```python
from build123d import *
from OCP.BRepFilletAPI import BRepFilletAPI_MakeChamfer

# Parameters (mm, degrees)
SKETCH1_W               = 71
SKETCH1_H               = 71
SKETCH1_W_2             = 21
SKETCH1_H_2             = 21
BOSS_EXTRUDE1_DEPTH     = 25
SKETCH2_W               = 21
SKETCH2_H               = 23
BOSS_EXTRUDE2_DEPTH     = 2
CHAMFER1_SIZE           = 2
CHAMFER1_SIZE_2         = 20
CUT_EXTRUDE1_DEPTH      = 84.846586096
CUT_EXTRUDE1_DEPTH_BACK = 5
SKETCH3_R               = 1.5
SKETCH4_R               = 1.5
CUT_EXTRUDE2_DEPTH      = 5
CUT_EXTRUDE3_START      = -5
SKETCH5_R               = 1.5
CUT_EXTRUDE3_DEPTH      = 5
SKETCH6_W               = 21
SKETCH6_H               = 20
SKETCH6_R               = 2.5
CUT_EXTRUDE4_DEPTH      = 21
CUT_EXTRUDE5_DEPTH      = 30
CHAMFER2_SIZE           = 2


with BuildPart() as part:
    # Sketch1 → Boss-Extrude1 (new body)
    with BuildSketch(Plane(origin=(0, 0, 0), x_dir=(1, 0, 0), z_dir=(0, 1, 0))):
        Rectangle(SKETCH1_W, SKETCH1_H)
        Polygon((-13, 9.464466094), (-13, -9.464466094), (-30.5, -26.964466094), (-30.5, 26.964466094), align=None, mode=Mode.SUBTRACT)
        Rectangle(SKETCH1_W_2, SKETCH1_H_2, mode=Mode.SUBTRACT)
        Polygon((30.5, -26.964466094), (13, -9.464466094), (13, 9.464466094), (30.5, 26.964466094), align=None, mode=Mode.SUBTRACT)
        Polygon((9.464466094, 13), (-9.464466094, 13), (-26.964466094, 30.5), (26.964466094, 30.5), align=None, mode=Mode.SUBTRACT)
    extrude(amount=BOSS_EXTRUDE1_DEPTH)

    # Sketch2 → Boss-Extrude2 (add)
    with BuildSketch(Plane(origin=(0, 25, 0), x_dir=(1, 0, 0), z_dir=(0, 1, 0))):
        Polygon((-33.5, -35.5), (-10.5, -35.5), (-10.5, -12.5), align=None)
        with Locations((0, -24)):
            Rectangle(SKETCH2_W, SKETCH2_H)
        Polygon((10.5, -12.5), (10.5, -35.5), (33.5, -35.5), align=None)
    extrude(amount=BOSS_EXTRUDE2_DEPTH)

    # Chamfer1
    chamfer1_edges_1 = [part.edges().sort_by_distance(p)[0] for p in [
        (22, 27, 24),
    ]]
    chamfer1_side_1 = [part.faces().sort_by_distance(p)[0] for p in [
        (22, 26.96, 24),
    ]]
    chamfer1_edges_2 = [part.edges().sort_by_distance(p)[0] for p in [
        (0, 27, 12.5),
    ]]
    chamfer1_side_2 = [part.faces().sort_by_distance(p)[0] for p in [
        (0, 26.96, 12.5),
    ]]
    chamfer1_edges_3 = [part.edges().sort_by_distance(p)[0] for p in [
        (-22, 27, 24),
    ]]
    chamfer1_side_3 = [part.faces().sort_by_distance(p)[0] for p in [
        (-22, 26.96, 24),
    ]]
    chamfer1 = BRepFilletAPI_MakeChamfer(part.part.solid().wrapped)
    for e in chamfer1_edges_1:
        chamfer1.Add(CHAMFER1_SIZE - 0.0001, CHAMFER1_SIZE_2 - 0.0001, e.wrapped, chamfer1_side_1[0].wrapped)
    for e in chamfer1_edges_2:
        chamfer1.Add(CHAMFER1_SIZE - 0.0001, CHAMFER1_SIZE_2 - 0.0001, e.wrapped, chamfer1_side_2[0].wrapped)
    for e in chamfer1_edges_3:
        chamfer1.Add(CHAMFER1_SIZE - 0.0001, CHAMFER1_SIZE_2 - 0.0001, e.wrapped, chamfer1_side_3[0].wrapped)
    add(Compound.cast(chamfer1.Shape()), mode=Mode.REPLACE)  # a hair under: the kernel refuses the full size

    # Sketch3 → Cut-Extrude1 (cut, two sides: drawn at the far end of the back side and taken through both)
    with BuildSketch(Plane.ZY.offset(35.5).offset(-CUT_EXTRUDE1_DEPTH_BACK)):
        with Locations(Location((-10, 12.5, 0), (0, 0, 180))):
            Circle(SKETCH3_R)
        with BuildLine():
            ThreePointArc((0, 14), (-1.5, 12.5), (0, 11))
            Line((0, 11), (0, 14))
        make_face()
        with BuildLine():
            Line((0, 14), (0, 11))
            ThreePointArc((0, 11), (1.060660172, 11.439339828), (1.5, 12.5))
            ThreePointArc((1.5, 12.5), (1.060660172, 13.560660172), (0, 14))
        make_face()
        with Locations(Location((10, 12.5, 0), (0, 0, 180))):
            Circle(SKETCH3_R)
    extrude(amount=CUT_EXTRUDE1_DEPTH + CUT_EXTRUDE1_DEPTH_BACK, mode=Mode.SUBTRACT)

    # Sketch4 → Cut-Extrude2 (cut)
    with BuildSketch(Plane(origin=(0, 0, -35.5), x_dir=(-1, 0, 0), z_dir=(0, 0, -1))):
        with Locations((-10, 12.5)):
            Circle(SKETCH4_R)
        with Locations((0, 12.5)):
            Circle(SKETCH4_R)
        with Locations((10, 12.5)):
            Circle(SKETCH4_R)
    extrude(amount=-CUT_EXTRUDE2_DEPTH, mode=Mode.SUBTRACT)

    # Sketch5 → Cut-Extrude3 (cut)
    with BuildSketch(Plane(origin=(35.5, 0, 0), x_dir=(0, 0, -1), z_dir=(1, 0, 0)).offset(CUT_EXTRUDE3_START)):
        with Locations((-10, 12.5)):
            Circle(SKETCH5_R)
        with BuildLine():
            ThreePointArc((1.5, 12.5), (1.060660172, 13.560660172), (0, 14))
            Line((0, 14), (0, 11))
            ThreePointArc((0, 11), (1.060660172, 11.439339828), (1.5, 12.5))
        make_face()
        with BuildLine():
            Line((0, 11), (0, 14))
            ThreePointArc((0, 14), (-1.5, 12.5), (0, 11))
        make_face()
        with Locations((10, 12.5)):
            Circle(SKETCH5_R)
    extrude(amount=CUT_EXTRUDE3_DEPTH, mode=Mode.SUBTRACT)

    # Sketch6 → Cut-Extrude4 (cut)
    with BuildSketch(Plane.XY.offset(35.5)):
        with Locations((0, 10)):
            Rectangle(SKETCH6_W, SKETCH6_H)
        with Locations((0, 10)):
            Circle(SKETCH6_R, mode=Mode.SUBTRACT)
    extrude(amount=-CUT_EXTRUDE4_DEPTH, mode=Mode.SUBTRACT)

    # Sketch6<2> → Cut-Extrude5 (cut)
    with BuildSketch(Plane.XY.offset(35.5)):
        with BuildLine():
            ThreePointArc((0, 12.5), (-2.5, 10), (0, 7.5))
            Line((0, 7.5), (0, 12.5))
        make_face()
        with BuildLine():
            Line((0, 12.5), (0, 7.5))
            ThreePointArc((0, 7.5), (1.767766953, 8.232233047), (2.5, 10))
            ThreePointArc((2.5, 10), (1.767766953, 11.767766953), (0, 12.5))
        make_face()
    extrude(amount=-CUT_EXTRUDE5_DEPTH, mode=Mode.SUBTRACT)

    # Chamfer2
    chamfer2_edges = [part.edges().sort_by_distance(p)[0] for p in [
        (-18.214466094, 25, -21.75),
        (-30.5, 25, 0),
        (-21.75, 25, -18.214466094),
        (-21.75, 25, 18.214466094),
        (0, 25, -30.5),
        (30.5, 25, 0),
        (21.75, 25, 18.214466094),
        (18.214466094, 25, -21.75),
        (21.75, 25, -18.214466094),
    ]]
    chamfer(chamfer2_edges, length=CHAMFER2_SIZE)


solid = part.part
```
Part model, mm, in its own coordinate system. A direction names the side the tool comes from. Coordinates: 2 decimals unless noted, no trailing zeros. Loops run counter-clockwise (first coordinate to the right, second up) from the corner with the lowest first, then second, coordinate; pieces in that order, holes last. Notation, with made-up numbers: (5, 52.5) - (41, 52.5) arc R19 cw to (41, 87.5) - close; hole circle Ø2 at (-39.75, -4.75). An arc over 180 degrees is marked (long way). Write item = value, one per line. Start each with the question number.
Item 1: Cut at C-C, the plane x = -20.5. State how many separate pieces and enclosed holes the cut face has, and give its area (3 significant figures).
Item 2: 3-axis set-ups, long thin cutter, end or side, ignore diameter. For faces 5 (the flat face through (22.614, 23.986, -20.472)), 6 (the cylindrical face through (-32.97, 12.43, -8.5)), 7 (the flat face through (-2, 12, 10.5)), 8 (the flat face through (-2, 12, 14.5)): which of +Z, -Z, +X, -X, +Y, -Y reach the whole face in a straight line?
Item 3: Wall check: L1, parallel to Z at x = 2.5, y = 10.5; L2, parallel to X at y = 14.25, z = 25.5; L3, parallel to Z at x = -26.5, y = 11.5. Give the ranges that are in metal, low to high. Write a range as from..to.
Item 4: Flat gauge pins, fed straight in: pin 1 Ø10 at (x, y) = (-5, 8.5) entering from +Z; pin 2 Ø2.5 at (y, z) = (12.5, -10) entering from +X; pin 3 Ø6 at (x, z) = (-11.5, 19.5) entering from +Y. Where does each tip first touch, or does it go through?
Item 5: Cut at B-B, the plane y = 2. Give the cut face in (x, z).
Item 6: Cut at A-A, the plane z = -5. Give the cut face in (x, y), and give its area (3 significant figures).
Item 7: Cut at D-D, the plane z = -29. Give the cut face in (x, y), and give its area (3 significant figures).
Item 8: Mould opens along Z. For faces 1 (the flat face through (14.01, 25.79, 27.2)), 2 (the cylindrical face through (-8.5, 12.57, -33.03)), 3 (the flat face through (-21.872, 11.339, -18.337)), 4 (the flat face through (0, 22, 35.5)) say: released by +Z, released by -Z, zero draft, split by the parting line, or undercut.
The answers:
q1.separate_pieces = 3
q1.enclosed_holes = 0
q1.area = 761 mm2
q2.face_5 = +Y
q2.face_6 = -X
q2.face_7 = +Y, -Y
q2.face_8 = +Z, -Y
q3.L1 = -35.5..-30.5, -13..-10.5, 10.5..14.5
q3.L2 = -35.5..-30.5, -29.04..-10.5, 10.5..29.04, 30.5..35.5
q3.L3 = -35.5..-30.5, -30.04..-22.96, 22.96..35.5
q4.pin_1 = 14.5
q4.pin_2 = 14.79
q4.pin_3 = 25.72
q5.outline = (-35.5, -35.5) - (35.5, -35.5) - (35.5, 35.5) - (10.5, 35.5) - (10.5, 14.5) - (-10.5, 14.5) - (-10.5, 35.5) - (-35.5, 35.5) - close; hole (-30.5, -26.96) - (-13, -9.46) - (-13, 9.46) - (-30.5, 26.96) - close; hole (-26.96, -30.5) - (26.96, -30.5) - (9.46, -13) - (-9.46, -13) - close; hole (-10.5, -10.5) - (10.5, -10.5) - (10.5, 10.5) - (-10.5, 10.5) - close; hole (13, -9.46) - (30.5, -26.96) - (30.5, 26.96) - (13, 9.46) - close
q6.outline = (-35.5, 0) - (-30.5, 0) - (-30.5, 23) - (-32.5, 25) - (-35.5, 25) - close; (-13, 0) - (-10.5, 0) - (-10.5, 25) - (-13, 25) - close; (10.5, 0) - (13, 0) - (13, 25) - (10.5, 25) - close; (30.5, 0) - (35.5, 0) - (35.5, 25) - (32.5, 25) - (30.5, 23) - close
q6.area = 371 mm2
q7.outline = (-35.5, 0) - (-25.46, 0) - (-25.46, 23) - (-28.29, 25) - (-29.71, 25) - (-31.34, 23.84) - (-32.5, 25) - (-35.5, 25) - close; (25.46, 0) - (35.5, 0) - (35.5, 25) - (32.5, 25) - (31.34, 23.84) - (29.71, 25) - (28.29, 25) - (25.46, 23) - close
q7.area = 493 mm2
q8.face_1 = released by -Z
q8.face_2 = zero draft
q8.face_3 = undercut
q8.face_4 = released by +Z
